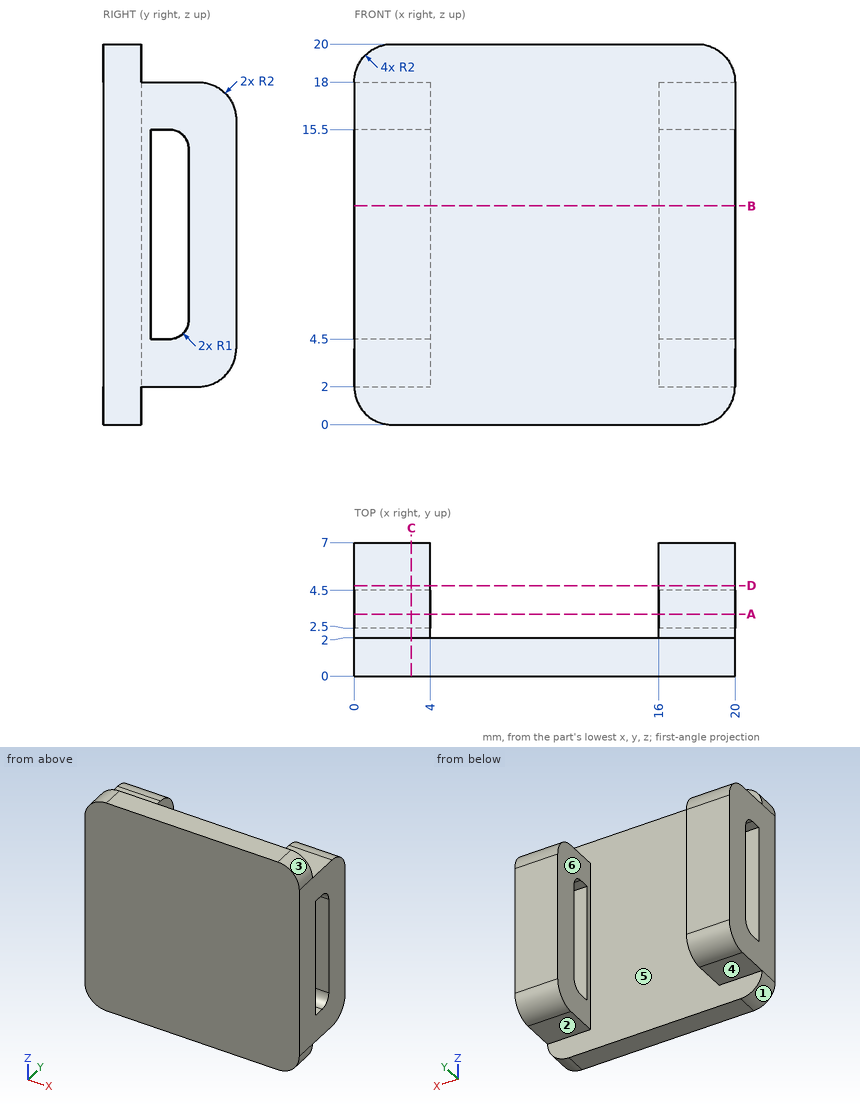
Design review of the part shown in the three views and the two pictorial views. Dimensions are in mm from the part's minimum x, y and z. A direction names the side the tool comes from. Round coordinates to 2 decimals unless told otherwise and drop trailing zeros. Loops run counter-clockwise (first coordinate to the right, second up) from the corner with the lowest first, then second, coordinate; pieces in that order, holes last. Notation, with made-up numbers: M 18.5,40 L 41.5,40 A29 ccw 41.5,79 Z; hole C 36,78 d3. An arc over 180 degrees is marked long. Write item = value, one per line.
Item 1: Take a section at C-C on x = 3. Write out the cut boundary in (y, z), then the cut area to 3 significant figures.
Return value:
outline = M 0,0 L 2,0 L 2,2 L 5,2 A2 ccw 7,4 L 7,16 A2 ccw 5,18 L 2,18 L 2,20 L 0,20 Z; hole M 2.5,4.5 L 3.5,4.5 A1 ccw 4.5,5.5 L 4.5,14.5 A1 ccw 3.5,15.5 L 2.5,15.5 Z
area = 96.7 mm2
Item 2: Take a section at B-B on z = 11.5. Write out the cut boundary in (x, y), then the cut area to 3 significant figures.
Return value:
outline = M 0,0 L 20,0 L 20,2.5 L 16,2.5 L 16,2 L 4,2 L 4,2.5 L 0,2.5 Z; M 0,4.5 L 4,4.5 L 4,7 L 0,7 Z; M 16,4.5 L 20,4.5 L 20,7 L 16,7 Z
area = 64.0 mm2
Item 3: Machinability: for the marked faces 1 and 2, which of the approach directions +Z, -Z, +X, -X, +Y, -Y give a long, thin tool a straight path to every point of the face, cutting with its end or side? Answer none if there is none.
Return value:
face_1 = -Z, -X, +Y, -Y
face_2 = -Z, +X, -X, +Y
Item 4: The part is to be moulded in two halves that separate along X. For the marked faces 3, 4, 5 and 6, say which applies: released by +X, released by -X, zero draft, split by the parting line, or undercut.
Return value:
face_3 = released by +X
face_4 = zero draft
face_5 = undercut
face_6 = undercut
Item 5: Insertion check: P1, Ø4, axis at x = 5.5, z = 3, coming from the +Y side; P2, Ø2.5, axis at x = 1.5, y = 4, coming from the -Z side; P3, Ø0.5, axis at x = 18, y = 3, coming from the +Z side; P4, Ø3, axis at x = 10.5, z = 10, coming from the +Y side. Each pin has a flat end and moves straight along its axis. Give the tip position at first contact, or say it passes through.
Return value:
P1 = 7
P2 = 2
P3 = 18
P4 = 2
Item 6: Take a section at D-D on y = 4.75. Write out the cut boundary in (x, z).
Return value:
outline = M 0,2 L 4,2 L 4,18 L 0,18 Z; M 16,2 L 20,2 L 20,18 L 16,18 Z
Item 7: Take a section at A-A on y = 3.25. Write out the cut boundary in (x, z), then the cut area to 3 significant figures.
Return value:
outline = M 0,2 L 4,2 L 4,4.5 L 0,4.5 Z; M 0,15.5 L 4,15.5 L 4,18 L 0,18 Z; M 16,2 L 20,2 L 20,4.5 L 16,4.5 Z; M 16,15.5 L 20,15.5 L 20,18 L 16,18 Z
area = 40.0 mm2
Item 8: For line 1 (X direction, y = 5.5, z = 5.25); line 2 (Z direction, x = 1.5, y = 3); line 3 (Y direction, x = 3.75, z = 13.5), list the stretches that pass through material, from the lowest coordinate up. Write a range as [from, to].
Return value:
line_1 = [0, 4], [16, 20]
line_2 = [2, 4.5], [15.5, 18]
line_3 = [0, 2.5], [4.5, 7]
